Build history of the part. All positions in model axes, mm. Coordinates: 2 decimals unless noted, no trailing zeros. Order: outer loops, then holes, each group sorted by start corner. A loop starts at its lowest first (then second) coordinate and runs counter-clockwise, first axis right, second up. Notation, with made-up numbers: (9.5, 52.5) - (66.5, 52.5) arc R25 ccw to (66.5, 75.5) - close; hole circle Ø1 at (4, 56). An arc over 180 degrees is marked (long way). Answer as CSV lines item,"result". Start each with the question number.
from build123d import *

# Parameters (mm, degrees)
F0_W     = 7
F0_H     = 70
F1_DEPTH = 8
F2_SIZE  = 6
F3_R     = 1.25
F4_DEPTH = 2.7
F5_R     = 1.25
F6_DEPTH = 2.7
F5_W     = 0.2
F5_H     = 0.5
F7_DEPTH = 0.15


with BuildPart() as f1:
    # F0 (on Top) → F1 (new body)
    with BuildSketch(Plane.XY):
        with Locations((-11.251043, -3.17281)):
            Rectangle(F0_W, F0_H)
    extrude(amount=F1_DEPTH)

    # F2
    f2_edges = [f1.edges().sort_by_distance(p)[0] for p in [
        (-14.751043, -3.17281, 8),
    ]]
    chamfer(f2_edges, length=F2_SIZE)

    # F3 (on face) → F4 (cut)
    with BuildSketch(Plane.YZ.offset(-7.751043)):
        with BuildLine():
            ThreePointArc((-23.17281, 2.75), (-22.288927, 3.116117), (-21.92281, 4))
            ThreePointArc((-21.92281, 4), (-24.056694, 4.883883), (-23.17281, 2.75))
        make_face()
        with Locations((-3.17281, 4)):
            Circle(F3_R)
        with BuildLine():
            ThreePointArc((16.82719, 2.75), (17.711073, 3.116117), (18.07719, 4))
            ThreePointArc((18.07719, 4), (15.943306, 4.883883), (16.82719, 2.75))
        make_face()
    extrude(amount=-F4_DEPTH, mode=Mode.SUBTRACT)

    # F5 (on face) → F6 (cut)
    with BuildSketch(Plane(origin=(0, 0, 0), x_dir=(1, 0, 0), z_dir=(0, 0, -1))):
        with Locations((-11.751043, -16.82719)):
            Circle(F5_R)
        with Locations((-11.751043, 3.17281)):
            Circle(F5_R)
        with Locations((-11.751043, 23.17281)):
            Circle(F5_R)
    extrude(amount=-F6_DEPTH, mode=Mode.SUBTRACT)

    # F5 (on face) → F7 (cut)
    with BuildSketch(Plane(origin=(0, 0, 0), x_dir=(1, 0, 0), z_dir=(0, 0, -1))):
        with Locations((-11.851043, -12.07719)):
            Rectangle(F5_W, F5_H)
    extrude(amount=-F7_DEPTH, mode=Mode.SUBTRACT)


solid = f1.part
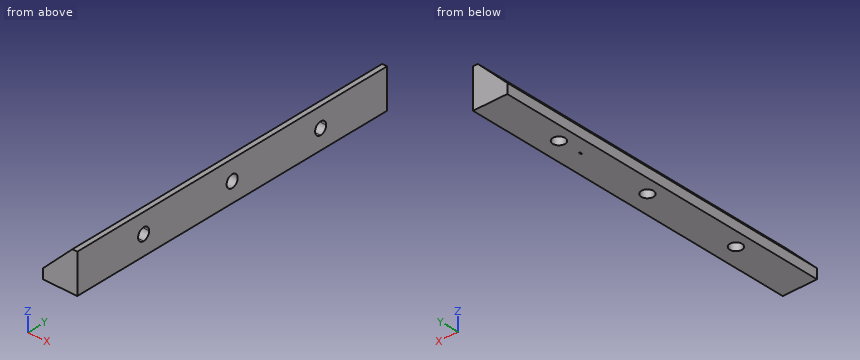
(1) Band-saw the part on C-C on x = -9.75. List the corners of the cut face in (y, z), plus the area to 3 significant figures.
(2) Probe L1, parallel to Y at x = -8, z = 3; L2, parallel to Y at x = -11.5, z = 1.5; L3, parallel to X at y = -12, z = 5. List the from-to ranges inside material, lowest first. Write a range as [from, to].
(3) Band-saw the part on D-D on z = 6.5. List the corners of the cut face in (x, y).
(4) Band-saw the part on B-B on y = -25. List the corners of the cut face in (x, z), plus the area to 3 significant figures.
(5) Drop flat-ended pins along their axis: pin 1 Ø0.8 at (x, y) = (-11.5, -2.5) entering from -Z; pin 2 Ø1.2 at (y, z) = (-3.5, 3.5) entering from +X; pin 3 Ø3 at (y, z) = (-3.17, 4) entering from +X; pin 4 Ø1.5 at (x, y) = (-11.5, -2.5) entering from +Z. Give the stop position or say it passes through.
(6) Band-saw the part on A-A on z = 1. List the corners of the cut face in (x, y).
Filled in:
1,outline,"(-38.17, 0) - (31.83, 0) - (31.83, 7) - (-38.17, 7) - close; hole (-23.17, 2.75) arc R1.25 ccw to (-21.92, 4) arc R1.25 ccw (long way) to start; hole circle Ø2.5 at (-3.17, 4); hole (16.83, 2.75) arc R1.25 ccw to (18.08, 4) arc R1.25 ccw (long way) to start"
1,area,"475 mm^2"
2,L1,"y = [-38.17, -23.92], [-22.42, -3.92], [-2.42, 16.08], [17.58, 31.83]"
2,L2,"y = [-38.17, -24.4], [-21.95, -4.4], [-1.95, 15.6], [18.05, 31.83]"
2,L3,"x = [-11.75, -7.75]"
3,outline,"(-10.25, -38.17) - (-7.75, -38.17) - (-7.75, 31.83) - (-10.25, 31.83) - close"
4,outline,"(-14.75, 0) - (-7.75, 0) - (-7.75, 8) - (-8.75, 8) - (-14.75, 2) - close"
4,area,"38.0 mm^2"
5,pin 1,"stops at z = 2.7"
5,pin 2,"stops at x = -10.45"
5,pin 3,"stops at x = -7.75"
5,pin 4,"stops at z = 6"
6,outline,"(-14.75, -38.17) - (-7.75, -38.17) - (-7.75, 31.83) - (-14.75, 31.83) - close; hole circle Ø2.5 at (-11.75, -23.17); hole circle Ø2.5 at (-11.75, -3.17); hole circle Ø2.5 at (-11.75, 16.83)"
